from build123d import *

# Parameters (mm, degrees)
BOSS_EXTRUDE1_DEPTH = 2
BOSS_EXTRUDE2_DEPTH = 4
BOSS_EXTRUDE3_DEPTH = 4
SKETCH3_R           = 8.5
FORSENSORS_DEPTH    = 5
FORCRYSTAL_DEPTH    = 1
PCBLEDGE_DEPTH      = 0.5
GROOVE_DEPTH        = 2
SKETCH7_W           = 13.4
SKETCH7_H           = 2
BOSS_EXTRUDE5_DEPTH = 2


with BuildPart() as part:
    # Sketch1 → Boss-Extrude1 (new body)
    with BuildSketch(Plane(origin=(0, 0, 0), x_dir=(1, 0, 0), z_dir=(0, 1, 0))):
        Polygon((7, 12.5), (-23, 12.5), (-25, 10.5), (-25, -10.5), (-23, -12.5), (23, -12.5), (25, -10.5), (25, 10.5), (23, 12.5), align=None)
    extrude(amount=BOSS_EXTRUDE1_DEPTH)

    # Sketch2 → Boss-Extrude2 (add)
    with BuildSketch(Plane(origin=(0, 2, 0), x_dir=(1, 0, 0), z_dir=(0, 1, 0))):
        with BuildLine():
            Line((-19.25, 8.75), (-19.25, 10.5))
            Line((-19.25, 10.5), (-22.171572875, 10.5))
            Line((-22.171572875, 10.5), (-23, 9.671572875))
            Line((-23, 9.671572875), (-23, 7))
            Line((-23, 7), (-21, 7))
            ThreePointArc((-21, 7), (-19.762563133, 7.512563133), (-19.25, 8.75))
        make_face()
        with BuildLine():
            Line((22.171572875, 10.5), (19.25, 10.5))
            Line((19.25, 10.5), (19.25, 8.75))
            ThreePointArc((19.25, 8.75), (19.762563133, 7.512563133), (21, 7))
            Line((21, 7), (23, 7))
            Line((23, 7), (23, 9.671572875))
            Line((23, 9.671572875), (22.171572875, 10.5))
        make_face()
        with BuildLine():
            Line((-21, -7), (-23, -7))
            Line((-23, -7), (-23, -9.671572875))
            Line((-23, -9.671572875), (-22.171572875, -10.5))
            Line((-22.171572875, -10.5), (-19.25, -10.5))
            Line((-19.25, -10.5), (-19.25, -8.75))
            ThreePointArc((-19.25, -8.75), (-19.762563133, -7.512563133), (-21, -7))
        make_face()
        with BuildLine():
            Line((23, -9.671572875), (23, -7))
            Line((23, -7), (21, -7))
            ThreePointArc((21, -7), (19.762563133, -7.512563133), (19.25, -8.75))
            Line((19.25, -8.75), (19.25, -10.5))
            Line((19.25, -10.5), (22.171572875, -10.5))
            Line((22.171572875, -10.5), (23, -9.671572875))
        make_face()
    extrude(amount=BOSS_EXTRUDE2_DEPTH)

    # Sketch2_3 → Boss-Extrude3 (add)
    with BuildSketch(Plane(origin=(0, 2, 0), x_dir=(1, 0, 0), z_dir=(0, 1, 0))):
        Polygon((23, 12.5), (7.5, 12.5), (-7.5, 12.5), (-23, 12.5), (-25, 10.5), (-25, -10.5), (-23, -12.5), (0, -12.5), (23, -12.5), (25, -10.5), (25, 10.5), align=None)
        Polygon((-19.25, 10.5), (-1.449649569, 10.5), (1.449649569, 10.5), (19.25, 10.5), (22.171572875, 10.5), (23, 9.671572875), (23, 7), (23, -7), (23, -9.671572875), (22.171572875, -10.5), (19.25, -10.5), (0, -10.5), (-19.25, -10.5), (-22.171572875, -10.5), (-23, -9.671572875), (-23, -7), (-23, 7), (-23, 9.671572875), (-22.171572875, 10.5), align=None, mode=Mode.SUBTRACT)
    extrude(amount=BOSS_EXTRUDE3_DEPTH)

    # Sketch3 → ForSensors (cut)
    with BuildSketch(Plane.XZ):
        with Locations(Location((-13, 0, 0), (0, 0, 270))):
            Circle(SKETCH3_R)
        with Locations(Location((13, 0, 0), (0, 0, 270))):
            Circle(SKETCH3_R)
    extrude(amount=-FORSENSORS_DEPTH, mode=Mode.SUBTRACT)

    # Sketch4 → ForCrystal (cut)
    with BuildSketch(Plane(origin=(0, 2, 0), x_dir=(1, 0, 0), z_dir=(0, 1, 0))):
        with BuildLine():
            Line((3.9, -9.2), (-3.9, -9.2))
            ThreePointArc((-3.9, -9.2), (-6, -7.1), (-3.9, -5))
            Line((-3.9, -5), (3.9, -5))
            ThreePointArc((3.9, -5), (6, -7.1), (3.9, -9.2))
        make_face()
    extrude(amount=-FORCRYSTAL_DEPTH, mode=Mode.SUBTRACT)

    # Sketch5 → PcbLedge (add)
    with BuildSketch(Plane(origin=(0, 6, 0), x_dir=(1, 0, 0), z_dir=(0, 1, 0))):
        with BuildLine():
            ThreePointArc((-21, 7), (-19.762563133, 7.512563133), (-19.25, 8.75))
            Line((-19.25, 8.75), (-19.25, 10.2))
            Line((-19.25, 10.2), (-22.188730163, 10.2))
            Line((-22.188730163, 10.2), (-22.7, 9.688730163))
            Line((-22.7, 9.688730163), (-22.7, 7))
            Line((-22.7, 7), (-21, 7))
        make_face()
        with BuildLine():
            Line((-19.25, -10.2), (-19.25, -8.75))
            ThreePointArc((-19.25, -8.75), (-19.762563133, -7.512563133), (-21, -7))
            Line((-21, -7), (-22.7, -7))
            Line((-22.7, -7), (-22.7, -9.688730163))
            Line((-22.7, -9.688730163), (-22.188730163, -10.2))
            Line((-22.188730163, -10.2), (-19.25, -10.2))
        make_face()
        with BuildLine():
            ThreePointArc((19.25, 8.75), (19.762563133, 7.512563133), (21, 7))
            Line((21, 7), (22.7, 7))
            Line((22.7, 7), (22.7, 9.688730163))
            Line((22.7, 9.688730163), (22.188730163, 10.2))
            Line((22.188730163, 10.2), (19.25, 10.2))
            Line((19.25, 10.2), (19.25, 8.75))
        make_face()
        with BuildLine():
            Line((22.7, -7), (21, -7))
            ThreePointArc((21, -7), (19.762563133, -7.512563133), (19.25, -8.75))
            Line((19.25, -8.75), (19.25, -10.2))
            Line((19.25, -10.2), (22.188730163, -10.2))
            Line((22.188730163, -10.2), (22.7, -9.688730163))
            Line((22.7, -9.688730163), (22.7, -7))
        make_face()
    extrude(amount=PCBLEDGE_DEPTH)

    # Sketch6 → Groove (cut)
    with BuildSketch(Plane(origin=(0, 6, 0), x_dir=(1, 0, 0), z_dir=(0, 1, 0))):
        Polygon((25, 10.5), (23, 12.5), (6.7, 12.5), (6.7, 11.3), (22.502943725, 11.3), (23.8, 10.002943725), (23.8, -10.002943725), (22.502943725, -11.3), (-22.502943725, -11.3), (-23.8, -10.002943725), (-23.8, 10.002943725), (-22.502943725, 11.3), (-6.7, 11.3), (-6.7, 12.5), (-23, 12.5), (-25, 10.5), (-25, -10.5), (-23, -12.5), (23, -12.5), (25, -10.5), align=None)
    extrude(amount=-GROOVE_DEPTH, mode=Mode.SUBTRACT)

    # Sketch7 → Boss-Extrude5 (add)
    with BuildSketch(Plane(origin=(0, 6, 0), x_dir=(1, 0, 0), z_dir=(0, 1, 0))):
        with Locations((0, 11.5)):
            Rectangle(SKETCH7_W, SKETCH7_H)
    extrude(amount=BOSS_EXTRUDE5_DEPTH)


solid = part.part
Part model, mm, in its own coordinate system. A direction names the side the tool comes from. Coordinates: 2 decimals unless noted, no trailing zeros. Order: outer loops, then holes, each group sorted by start corner. A loop starts at its lowest first (then second) coordinate and runs counter-clockwise, first axis right, second up. Notation, with made-up numbers: M -14.5,-9.75 L -6.5,-9.75 A37 ccw -6.5,29.25 Z; hole C 82.25,21 d4. An arc over 180 degrees is marked long. Use a Markdown table: item, result.
(1) Cut at A-A on y = 5.5. Write the cut outline in (x, z), then the cut area to 3 significant figures.
A:
| item | result |
|---|---|
| outline | M -23.8,-10 L -22.5,-11.3 L -6.7,-11.3 L -6.7,-12.5 L 6.7,-12.5 L 6.7,-11.3 L 22.5,-11.3 L 23.8,-10 L 23.8,10 L 22.5,11.3 L -22.5,11.3 L -23.8,10 Z; hole M -23,-7 L -21,-7 A1.75 cw -19.25,-8.75 L -19.25,-10.5 L 19.25,-10.5 L 19.25,-8.75 A1.75 cw 21,-7 L 23,-7 L 23,7 L 21,7 A1.75 cw 19.25,8.75 L 19.25,10.5 L -19.25,10.5 L -19.25,8.75 A1.75 cw -21,7 L -23,7 Z |
| area | 172 mm^2 |
(2) Probe L1, parallel to X at y = 1, z = 0; L2, parallel to Z at x = -9, y = 4.5; L3, parallel to Z at x = 9.5, y = 2.5. List the from-to ranges inside material, lowest first.
A:
| item | result |
|---|---|
| L1 | x = -25 to -21.5, -4.5 to 4.5, 21.5 to 25 |
| L2 | z = -11.3 to -10.5, 10.5 to 11.3 |
| L3 | z = -12.5 to -10.5, 10.5 to 12.5 |
(3) Tool access for faces 1 (the flat face through (23.142, 5.014, -10.661)), 2 (the flat face through (-15, 5, -11.3)), 3 (the flat face through (-19.25, 4, -10)): list every direction of +Z, -Z, +X, -X, +Y, -Y with a clear straight run to the whole face (end or side of a thin tool).
A:
| item | result |
|---|---|
| face 1 | -Z, +X, +Y |
| face 2 | -Z, -X, +Y |
| face 3 | +Y |
(4) Pull direction X, two halves, no side cores. Call faces 4 (the cylindrical face through (19.776, 4.219, 7.499)), 5 (the flat face through (22, 4, 7)), 6 (the flat face through (0, 5, 11.3)), 7 (the flat face through (24, 2, 11.5)): released by +X, released by -X, zero draft, split by the parting line, or undercut.
A:
| item | result |
|---|---|
| face 4 | undercut |
| face 5 | undercut |
| face 6 | zero draft |
| face 7 | released by +X |
(5) Cut at D-D on z = -1.75. Write the cut outline in (x, y).
A:
| item | result |
|---|---|
| outline | M -25,0 L -21.32,0 L -21.32,2 L -23,2 L -23,6 L -23.8,6 L -23.8,4 L -25,4 Z; M -4.68,0 L 4.68,0 L 4.68,2 L -4.68,2 Z; M 21.32,0 L 25,0 L 25,4 L 23.8,4 L 23.8,6 L 23,6 L 23,2 L 21.32,2 Z |
(6) Flat gauge pins, fed straight in: pin 1 (3.5 mm diameter, centred on x = -20.5, z = -9, fed in from +Y); pin 2 (0.6 mm diameter, centred on x = -22, y = 5.5, fed in from +Z); pin 3 (3 mm diameter, centred on y = 7, z = 2, fed in from -X). Where does each tip first touch, or does it go through?
A:
| item | result |
|---|---|
| pin 1 | stops at y = 6.5 |
| pin 2 | stops at z = 11.3 |
| pin 3 | stops at x = -23.8 |
(7) Cut at B-B on z = 6.5. Write the cut outline in (x, y).
A:
| item | result |
|---|---|
| outline | M -25,0 L -18.48,0 L -18.48,2 L -23,2 L -23,6 L -23.8,6 L -23.8,4 L -25,4 Z; M -7.52,0 L 7.52,0 L 7.52,2 L 5.91,2 L 5.91,1 L -5.91,1 L -5.91,2 L -7.52,2 Z; M 18.48,0 L 25,0 L 25,4 L 23.8,4 L 23.8,6 L 23,6 L 23,2 L 18.48,2 Z |
(8) Cut at C-C on x = 13. Write the cut outline in (y, z), then the cut area to 3 significant figures.
A:
| item | result |
|---|---|
| outline | M 0,-12.5 L 4,-12.5 L 4,-11.3 L 6,-11.3 L 6,-10.5 L 2,-10.5 L 2,-8.5 L 0,-8.5 Z; M 0,8.5 L 2,8.5 L 2,10.5 L 6,10.5 L 6,11.3 L 4,11.3 L 4,12.5 L 0,12.5 Z |
| area | 27.2 mm^2 |
